Geometry: final body of the model. Coordinates: model frame, mm. Round coordinates to 2 decimals unless told otherwise and drop trailing zeros. Write each loop counter-clockwise with the first axis right and the second up, starting at its lowest first coordinate (ties: lowest second). Pieces come first, ordered by that corner, then holes. Notation, with made-up numbers: M -16,70.5 L 36,70.5 A22 cw 36,93.5 Z; hole C -24,1 d8. An arc over 180 degrees is marked long. Use one line per item in the form item = value. Start each with the question number.
Item 1: Ray query, probe 1 along X at (y, z) = (3.7, 35.5); probe 2 along Z at (x, y) = (-80, 4.35); probe 3 along X at (y, z) = (2.75, 60). Return the intervals inside material, ascending.
Item 2: Section query A-A (x = -62). Return loops of the section in (y, z).
Item 3: Section query C-C (x = -108). Return loops of the section in (y, z), and give its area (3 significant figures).
Item 4: Section query D-D (z = -60). Return loops of the section in (x, y), and give its area (3 significant figures).
Item 5: Section query B-B (z = -15.5). Return loops of the section in (x, y).
from build123d import *

# Parameters (mm, degrees)
SKETCH_1_W                       = 236
SKETCH_1_H                       = 140
EXTRUDE_1_DEPTH                  = 5
CUT_EXTRUDE_1_REACH              = 139.292
SKETCH_2_W                       = 20
SKETCH_2_H                       = 5
PATTERN_LINEAR_1_COUNT           = 3
PATTERN_LINEAR_1_PITCH           = 40
PATTERN_LINEAR_2_COUNT           = 3
PATTERN_LINEAR_2_PITCH           = 40
CUT_EXTRUDE_2_REACH              = 139.292
SKETCH_3_W                       = 5
SKETCH_3_H                       = 25
PATTERN_LINEAR_6_COUNT           = 2
PATTERN_LINEAR_6_PITCH           = 75
PATTERN_LINEAR_6_COPY_1_REACH    = 139.292
PATTERN_LINEAR_6_COPY_1_SKETCH_W = 20
PATTERN_LINEAR_6_COPY_1_SKETCH_H = 5
PATTERN_LINEAR_6_COPY_2_REACH    = 139.292
PATTERN_LINEAR_6_COPY_2_SKETCH_W = 20
PATTERN_LINEAR_6_COPY_2_SKETCH_H = 5
PATTERN_LINEAR_6_COPY_3_REACH    = 139.292
PATTERN_LINEAR_6_COPY_3_SKETCH_W = 20
PATTERN_LINEAR_6_COPY_3_SKETCH_H = 5
PATTERN_LINEAR_6_COPY_4_REACH    = 139.292
PATTERN_LINEAR_6_COPY_4_SKETCH_W = 20
PATTERN_LINEAR_6_COPY_4_SKETCH_H = 5
PATTERN_LINEAR_7_COUNT           = 2
PATTERN_LINEAR_7_PITCH           = 45
PATTERN_LINEAR_7_COPY_1_REACH    = 139.292
PATTERN_LINEAR_7_COPY_1_SKETCH_W = 5
PATTERN_LINEAR_7_COPY_1_SKETCH_H = 25
SKETCH_4_R                       = 2.5
CUT_EXTRUDE_3_DEPTH              = 10


with BuildPart() as part:
    # 스케치1 → 보스-돌출1 (new body)
    with BuildSketch(Plane(origin=(0, 0, 0), x_dir=(1, 0, 0), z_dir=(0, 1, 0))):
        Rectangle(SKETCH_1_W, SKETCH_1_H)
    extrude(amount=EXTRUDE_1_DEPTH)

    # 스케치2 → 컷-돌출1 (cut, up to next)
    with BuildSketch(Plane(origin=(0, 5, 0), x_dir=(1, 0, 0), z_dir=(0, 1, 0)), mode=Mode.PRIVATE) as cut_extrude_1_sk1:
        with Locations((0, -42.5)):
            Rectangle(SKETCH_2_W, SKETCH_2_H)
    cut_extrude_1_tool1 = extrude(cut_extrude_1_sk1.sketch, amount=-CUT_EXTRUDE_1_REACH, mode=Mode.PRIVATE) & part.part
    cut_extrude_1 = cut_extrude_1_tool1.solids().sort_by_distance((0, 5, 42.5))[0]
    add(cut_extrude_1, mode=Mode.SUBTRACT)

    # 선형 패턴1: 컷-돌출1 ×3
    with Locations(*[(i * PATTERN_LINEAR_1_PITCH, 0, 0) for i in range(1, PATTERN_LINEAR_1_COUNT)]):
        add(cut_extrude_1, mode=Mode.SUBTRACT)

    # 선형 패턴2: 컷-돌출1 ×3
    with Locations(*[(-i * PATTERN_LINEAR_2_PITCH, 0, 0) for i in range(1, PATTERN_LINEAR_2_COUNT)]):
        add(cut_extrude_1, mode=Mode.SUBTRACT)

    # 스케치3 → 컷-돌출2 (cut, up to next)
    with BuildSketch(Plane(origin=(0, 5, 0), x_dir=(1, 0, 0), z_dir=(0, 1, 0)), mode=Mode.PRIVATE) as cut_extrude_2_sk1:
        with Locations((95.5, -27.5)):
            Rectangle(SKETCH_3_W, SKETCH_3_H)
    cut_extrude_2_tool1 = extrude(cut_extrude_2_sk1.sketch, amount=-CUT_EXTRUDE_2_REACH, mode=Mode.PRIVATE) & part.part
    cut_extrude_2 = cut_extrude_2_tool1.solids().sort_by_distance((95.5, 5, 27.5))[0]
    add(cut_extrude_2, mode=Mode.SUBTRACT)

    # 대칭 복사3: 컷-돌출2 across plane
    add(cut_extrude_2.mirror(Plane(origin=(0, 0, 0), x_dir=(0, 0, 1), z_dir=(1, 0, 0))), mode=Mode.SUBTRACT)

    # 선형 패턴6: 컷-돌출1 ×2
    with Locations(*[(0, 0, -i * PATTERN_LINEAR_6_PITCH) for i in range(1, PATTERN_LINEAR_6_COUNT)]):
        add(cut_extrude_1, mode=Mode.SUBTRACT)

    # 선형 패턴6 copy 1 sketch → 선형 패턴6 copy 1 (cut, up to next)
    with BuildSketch(Plane(origin=(40, 5, -75), x_dir=(1, 0, 0), z_dir=(0, 1, 0)), mode=Mode.PRIVATE) as pattern_linear_6_copy_1_sk1:
        with Locations((0, -42.5)):
            Rectangle(PATTERN_LINEAR_6_COPY_1_SKETCH_W, PATTERN_LINEAR_6_COPY_1_SKETCH_H)
    pattern_linear_6_copy_1_tool1 = extrude(pattern_linear_6_copy_1_sk1.sketch, amount=-PATTERN_LINEAR_6_COPY_1_REACH, mode=Mode.PRIVATE) & part.part
    add(pattern_linear_6_copy_1_tool1.solids().sort_by_distance((40, 5, -32.5))[0], mode=Mode.SUBTRACT)

    # 선형 패턴6 copy 2 sketch → 선형 패턴6 copy 2 (cut, up to next)
    with BuildSketch(Plane(origin=(80, 5, -75), x_dir=(1, 0, 0), z_dir=(0, 1, 0)), mode=Mode.PRIVATE) as pattern_linear_6_copy_2_sk1:
        with Locations((0, -42.5)):
            Rectangle(PATTERN_LINEAR_6_COPY_2_SKETCH_W, PATTERN_LINEAR_6_COPY_2_SKETCH_H)
    pattern_linear_6_copy_2_tool1 = extrude(pattern_linear_6_copy_2_sk1.sketch, amount=-PATTERN_LINEAR_6_COPY_2_REACH, mode=Mode.PRIVATE) & part.part
    add(pattern_linear_6_copy_2_tool1.solids().sort_by_distance((80, 5, -32.5))[0], mode=Mode.SUBTRACT)

    # 선형 패턴6 copy 3 sketch → 선형 패턴6 copy 3 (cut, up to next)
    with BuildSketch(Plane(origin=(-40, 5, -75), x_dir=(1, 0, 0), z_dir=(0, 1, 0)), mode=Mode.PRIVATE) as pattern_linear_6_copy_3_sk1:
        with Locations((0, -42.5)):
            Rectangle(PATTERN_LINEAR_6_COPY_3_SKETCH_W, PATTERN_LINEAR_6_COPY_3_SKETCH_H)
    pattern_linear_6_copy_3_tool1 = extrude(pattern_linear_6_copy_3_sk1.sketch, amount=-PATTERN_LINEAR_6_COPY_3_REACH, mode=Mode.PRIVATE) & part.part
    add(pattern_linear_6_copy_3_tool1.solids().sort_by_distance((-40, 5, -32.5))[0], mode=Mode.SUBTRACT)

    # 선형 패턴6 copy 4 sketch → 선형 패턴6 copy 4 (cut, up to next)
    with BuildSketch(Plane(origin=(-80, 5, -75), x_dir=(1, 0, 0), z_dir=(0, 1, 0)), mode=Mode.PRIVATE) as pattern_linear_6_copy_4_sk1:
        with Locations((0, -42.5)):
            Rectangle(PATTERN_LINEAR_6_COPY_4_SKETCH_W, PATTERN_LINEAR_6_COPY_4_SKETCH_H)
    pattern_linear_6_copy_4_tool1 = extrude(pattern_linear_6_copy_4_sk1.sketch, amount=-PATTERN_LINEAR_6_COPY_4_REACH, mode=Mode.PRIVATE) & part.part
    add(pattern_linear_6_copy_4_tool1.solids().sort_by_distance((-80, 5, -32.5))[0], mode=Mode.SUBTRACT)

    # 선형 패턴7: 컷-돌출2 ×2
    with Locations(*[(0, 0, -i * PATTERN_LINEAR_7_PITCH) for i in range(1, PATTERN_LINEAR_7_COUNT)]):
        add(cut_extrude_2, mode=Mode.SUBTRACT)

    # 선형 패턴7 copy 1 sketch → 선형 패턴7 copy 1 (cut, up to next)
    with BuildSketch(Plane(origin=(0, 5, -45), x_dir=(-1, 0, 0), z_dir=(0, 1, 0)), mode=Mode.PRIVATE) as pattern_linear_7_copy_1_sk1:
        with Locations((95.5, 27.5)):
            Rectangle(PATTERN_LINEAR_7_COPY_1_SKETCH_W, PATTERN_LINEAR_7_COPY_1_SKETCH_H)
    pattern_linear_7_copy_1_tool1 = extrude(pattern_linear_7_copy_1_sk1.sketch, amount=-PATTERN_LINEAR_7_COPY_1_REACH, mode=Mode.PRIVATE) & part.part
    add(pattern_linear_7_copy_1_tool1.solids().sort_by_distance((-95.5, 5, -17.5))[0], mode=Mode.SUBTRACT)

    # 스케치4 → 컷-돌출3 (cut)
    with BuildSketch(Plane(origin=(0, 5, 0), x_dir=(1, 0, 0), z_dir=(0, 1, 0))):
        with Locations(Location((-108, 60, 0), (0, 0, 270))):
            Circle(SKETCH_4_R)
        with Locations(Location((108, -60, 0), (0, 0, 270))):
            Circle(SKETCH_4_R)
        with Locations(Location((-108, -60, 0), (0, 0, 270))):
            Circle(SKETCH_4_R)
        with Locations(Location((108, 60, 0), (0, 0, 270))):
            Circle(SKETCH_4_R)
        with Locations(Location((0, 60, 0), (0, 0, 270))):
            Circle(SKETCH_4_R)
        with Locations(Location((0, -60, 0), (0, 0, 270))):
            Circle(SKETCH_4_R)
        with Locations(Location((-62, 60, 0), (0, 0, 270))):
            Circle(SKETCH_4_R)
        with Locations(Location((56, 60, 0), (0, 0, 270))):
            Circle(SKETCH_4_R)
        with Locations(Location((-10, 60, 0), (0, 0, 270))):
            Circle(SKETCH_4_R)
    extrude(amount=-CUT_EXTRUDE_3_DEPTH, mode=Mode.SUBTRACT)


solid = part.part
Working result:
q1.probe_1 = -118 to -98, -93 to 93, 98 to 118
q1.probe_2 = -70 to -35, -30 to 40, 45 to 70
q1.probe_3 = -118 to -110.5, -105.5 to -2.5, 2.5 to 105.5, 110.5 to 118
q2.outline = M 0,-70 L 5,-70 L 5,-62.5 L 0,-62.5 Z; M 0,-57.5 L 5,-57.5 L 5,70 L 0,70 Z
q3.outline = M 0,-70 L 5,-70 L 5,-62.5 L 0,-62.5 Z; M 0,-57.5 L 5,-57.5 L 5,57.5 L 0,57.5 Z; M 0,62.5 L 5,62.5 L 5,70 L 0,70 Z
q3.area = 650 mm²
q4.outline = M -118,0 L -110.5,0 L -110.5,5 L -118,5 Z; M -105.5,0 L -64.5,0 L -64.5,5 L -105.5,5 Z; M -59.5,0 L -12.5,0 L -12.5,5 L -59.5,5 Z; M -7.5,0 L -2.5,0 L -2.5,5 L -7.5,5 Z; M 2.5,0 L 53.5,0 L 53.5,5 L 2.5,5 Z; M 58.5,0 L 105.5,0 L 105.5,5 L 58.5,5 Z; M 110.5,0 L 118,0 L 118,5 L 110.5,5 Z
q4.area = 1,030 mm²
q5.outline = M -118,0 L -98,0 L -98,5 L -118,5 Z; M -93,0 L 93,0 L 93,5 L -93,5 Z; M 98,0 L 118,0 L 118,5 L 98,5 Z
